from build123d import *

# Parameters (mm, degrees)
F0_R     = 50.8
F1_DEPTH = 5
F2_R     = 6.35
F3_DEPTH = 5.001
F5_SIZE  = 5.08


# Not quite as in the source:
# - a fillet or chamfer that OpenCascade refuses, or shapes differently, is made with other operations: its cross-section is extruded or revolved along the edge and cut away or added


with BuildPart() as f1:
    # F0 (on Top) → F1 (new body)
    with BuildSketch(Plane.XY):
        Circle(F0_R)
    extrude(amount=F1_DEPTH)

    # F2 (on face) → F3 (cut, through all)
    with BuildSketch(Plane.XY.offset(5)):
        Circle(F2_R)
    extrude(amount=-F3_DEPTH, mode=Mode.SUBTRACT)

    # F4: chamfer of 5.08 on 1 edges, made by hand

    # F4_s1 → F4_t2 (revolve, cut)
    with BuildSketch(Plane.XZ):
        Polygon((50.8, -0.08), (45.72, 5), (50.8, 5), align=None)
    revolve(axis=Axis((0, 0, 5), (0, 0, 1)), mode=Mode.SUBTRACT)

    # F5
    f5_edges = [f1.edges().sort_by_distance(p)[0] for p in [
        (-50.72, 0, 0),
    ]]
    chamfer(f5_edges, length=F5_SIZE)


solid = f1.part
For this review, take the finished solid that the model builds, in its own axes (mm). Coordinates: 2 decimals unless noted, no trailing zeros. Order: outer loops, then holes, each group sorted by start corner. A loop starts at its lowest first (then second) coordinate and runs counter-clockwise, first axis right, second up. Notation, with made-up numbers: (-35, -33) - (-24, -33) arc R15 ccw to (-24, -19) - close; hole circle Ø1 at (49.5, -37.75). An arc over 180 degrees is marked (long way). Answer as CSV lines item,"result". Start each with the question number.
1) Draft analysis for pull direction X (two halves, no side actions). For faces 1 (the conical face through (-9.914, -44.646, 0.225)), 2 (the flat face through (-1, -10, 0)), 3 (the cylindrical face through (-1.38, -6.2, 2.54)), state which applies: +X half, -X half, draft (parallel to the pull), parting line (faces both ways), or undercut.
2) Add section C-C (z = 1.45). State the section outline as (x, y) points, then the cut area to 3 significant figures.
3) Insertion check: P1, Ø1, axis at x = -7, z = 2, coming from the +Y side; P2, Ø3, axis at y = -5.5, z = 2.5, coming from the +X side; P3, Ø1, axis at x = -24, z = 3.5, coming from the -Y side. Each pin has a flat end and moves straight along its axis. Give the tip position at first contact, or say it passes through.
4) To check wall thickness, follow line 1 along X through (y, z) = (-3.5, 1.6); line 2 along Y through (x, z) = (-5, 0.75); line 3 along Y through (x, z) = (5, 2.7). State the ranges of each line that lie inside material, in increasing order. Write a range as [from, to].
5) Add section A-A (x = 0). State the section outline as (y, z) points, then the cut area to 3 significant figures.
Result:
1,face 1,"parting line"
1,face 2,"draft"
1,face 3,"undercut"
2,outline,"circle Ø92.48 at (0, 0); hole circle Ø12.7 at (0, 0)"
2,area,"6,590 mm^2"
3,P1,"y = 46.16"
3,P2,"x = 46.92"
3,P3,"y = -40.85"
4,line 1,"[-46.17, -5.3], [5.3, 46.17]"
4,line 2,"[-45.68, -3.91], [3.91, 45.68]"
4,line 3,"[-46.49, -3.91], [3.91, 46.49]"
5,outline,"(-47.13, 3.59) - (-45.64, 0) - (-6.35, 0) - (-6.35, 5) - (-45.72, 5) - close; (6.35, 0) - (45.64, 0) - (47.13, 3.59) - (45.72, 5) - (6.35, 5) - close"
5,area,"400 mm^2"
